The figure shows three views and two pictorial views of one solid part (mm, origin at its lowest corner). Answer the questions. Round coordinates to 2 decimals unless told otherwise and drop trailing zeros. Order: outer loops, then holes, each group sorted by start corner. A loop starts at its lowest first (then second) coordinate and runs counter-clockwise, first axis right, second up. Notation, with made-up numbers: (23.25, 54) -> (67.25, 54) arc R21 cw to (67.25, 85) -> close; hole circle Ø9 at (46.5, 25). An arc over 180 degrees is marked (long way). Answer in a Markdown table with one row per item. Add a question column.
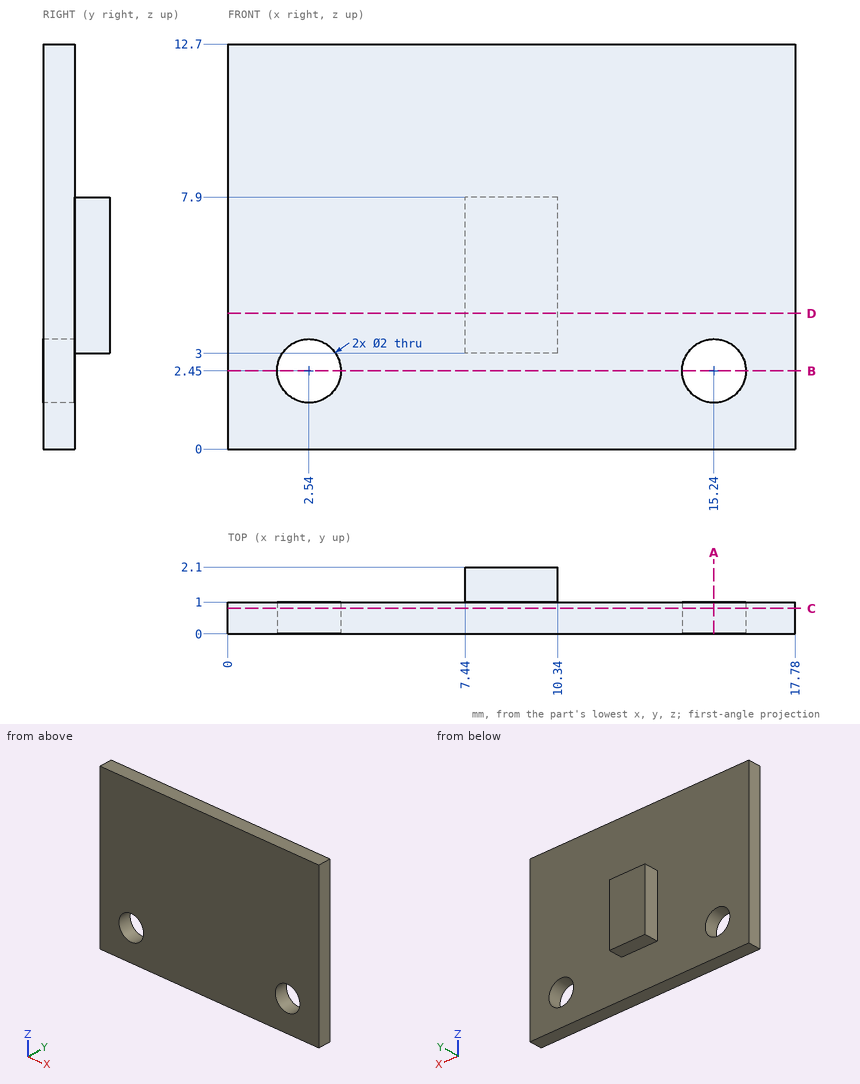
1. The part is cut by section C-C (y = 0.8). Give the vertices of the cut face in (x, z), then the cut area to 3 significant figures.
2. The part is cut by section D-D (z = 4.25). Give the vertices of the cut face in (x, y), then the cut area to 3 significant figures.
3. This flat-tipped pin is pushed along its axis until it touches: pin 1 (0.9 mm diameter, centred on y = 1.5, z = 6.5, fed in from -X). Where does it stop, or does it pass through?
4. Straight lines are drawn through the part: line 1 along X through (y, z) = (0.75, 2.45); line 2 along Y through (x, z) = (3.25, 8.25); line 3 along X through (y, z) = (1.4, 7). For each, find the intervals that lie inside material, in ascending order.
5. The part is cut by section B-B (z = 2.45). Give the vertices of the cut face in (x, y), then the cut area to 3 significant figures.
6. The part is cut by section A-A (x = 15.24). Give the vertices of the cut face in (y, z), then the cut area to 3 significant figures.
Report:
| question | item | result |
|---|---|---|
| 1 | outline | (0, 0) -> (17.78, 0) -> (17.78, 12.7) -> (0, 12.7) -> close; hole circle Ø2 at (2.54, 2.45); hole circle Ø2 at (15.24, 2.45) |
| 1 | area | 220 mm^2 |
| 2 | outline | (0, 0) -> (17.78, 0) -> (17.78, 1) -> (10.34, 1) -> (10.34, 2.1) -> (7.44, 2.1) -> (7.44, 1) -> (0, 1) -> close |
| 2 | area | 21.0 mm^2 |
| 3 | pin 1 | stops at x = 7.44 |
| 4 | line 1 | x = 0 to 1.54, 3.54 to 14.24, 16.24 to 17.78 |
| 4 | line 2 | y = 0 to 1 |
| 4 | line 3 | x = 7.44 to 10.34 |
| 5 | outline | (0, 0) -> (1.54, 0) -> (1.54, 1) -> (0, 1) -> close; (3.54, 0) -> (14.24, 0) -> (14.24, 1) -> (3.54, 1) -> close; (16.24, 0) -> (17.78, 0) -> (17.78, 1) -> (16.24, 1) -> close |
| 5 | area | 13.8 mm^2 |
| 6 | outline | (0, 0) -> (1, 0) -> (1, 1.45) -> (0, 1.45) -> close; (0, 3.45) -> (1, 3.45) -> (1, 12.7) -> (0, 12.7) -> close |
| 6 | area | 10.7 mm^2 |
